Autodesk Inventor part; units mm, degrees
ref_plane "YZ Plane" through (0, 0, 0) normal (1, 0, 0) x (0, 1, 0)
ref_plane "XZ Plane" through (0, 0, 0) normal (0, 1, 0) x (-1, 0, 0)
ref_plane "XY Plane" through (0, 0, 0) normal (0, 0, 1) x (1, 0, 0)
sketch "Sketch1" plane through (0, 0, 0) normal (0, 0, 1) x (1, 0, 0)
  arc A0 (-18.1959, 74.3045) -> (-75.755, 10.6506) centre (0, 0) ccw
  line L0 (-78.9841, -12.3172) -> (-75.755, 10.6506)
  arc A1 (12.2439, 58.7374) -> (-59.4846, -7.8472) centre (0, 0) ccw
  line L1 (-18.1959, 74.3045) -> (9.302, 81.0383)
  line L2 (-59.4846, -7.8472) -> (-58.6652, -14.0586)
  line L3 (-78.9841, -12.3172) -> (-58.6652, -14.0586)
  line L4 (12.2439, 58.7374) -> (9.302, 81.0383)
  circle A2 centre (-67.5, 0) radius 3
  circle A3 centre (0, 67.5) radius 3
  circle A4 centre (52.0914, 68.8152) radius 17.05 construction
  line L5 (-32.9083, 50.1702) -> (-43.208, 63.1294) construction
  line L6 (-50.5977, 32.2471) -> (-61.3205, 45.7388) construction
  circle A5 centre (-61.4614, 29.8439) radius 2.5
  circle A6 centre (-29.2318, 61.6164) radius 2.5
  point P0 (0, 0)
  dimension "d2" = 25
  dimension "d3" = 5
  dimension "d4" = 5
  dimension "d6" = 10
extrude "Extrusion1" add sketch "Sketch1" along normal blind 4.4
properties part number "FrontMotorPlateBridge"
Geometry: final body of the model. Coordinates: model frame, mm. A direction names the side the tool comes from. Coordinates: 2 decimals unless noted, no trailing zeros. Order: outer loops, then holes, each group sorted by start corner. A loop starts at its lowest first (then second) coordinate and runs counter-clockwise, first axis right, second up. Notation, with made-up numbers: (-14.5, -7) -> (0.5, -7) arc R31 ccw to (0.5, 26) -> close; hole circle Ø10 at (77, -29). An arc over 180 degrees is marked (long way). Use CSV: the item, a comma, the result in double quotes.
1) Section B-B on x = 0. Output: boundary loops of the cut face in (y, z).
Findings:
outline,"(60, 0) -> (64.5, 0) -> (64.5, 4.4) -> (60, 4.4) -> close; (70.5, 0) -> (78.76, 0) -> (78.76, 4.4) -> (70.5, 4.4) -> close"
2) Section D-D on y = 49. Output: boundary loops of the cut face in (x, z).
Findings:
outline,"(-58.75, 0) -> (-34.63, 0) -> (-34.63, 4.4) -> (-58.75, 4.4) -> close"
3) Line query: line 1 (X direction, y = 1, z = 2.35); line 2 (Y direction, x = -68, z = 3.55); line 3 (Y direction, x = 2, z = 3.1). Output: solid intervals per line, ascending.
Findings:
line 1,"x = -77.11 to -70.33, -64.67 to -59.99"
line 2,"y = -13.26 to -2.96, 2.96 to 35.05"
line 3,"y = 59.97 to 65.26, 69.74 to 79.25"
4) Section A-A on y = 0. Output: boundary loops of the cut face in (x, z), then the cut area to 3 significant figures.
Findings:
outline,"(-77.25, 0) -> (-70.5, 0) -> (-70.5, 4.4) -> (-77.25, 4.4) -> close; (-64.5, 0) -> (-60, 0) -> (-60, 4.4) -> (-64.5, 4.4) -> close"
area,"49.5 mm^2"
5) Section C-C on z = 3.3. Output: boundary loops of the cut face in (x, y) (1 decimal).
Findings:
outline,"(-79, -12.3) -> (-58.7, -14.1) -> (-59.5, -7.8) arc R60 cw to (12.2, 58.7) -> (9.3, 81) -> (-18.2, 74.3) arc R76.5 ccw to (-75.8, 10.7) -> close; hole circle Ø6 at (-67.5, 0); hole circle Ø5 at (-61.5, 29.8); hole circle Ø5 at (-29.2, 61.6); hole circle Ø6 at (0, 67.5)"
6) Pin query (flat end, axial travel): pin 1 Ø5 at (x, y) = (-67.5, 0) entering from +Z; pin 2 Ø1.5 at (x, z) = (-10.5, 2.5) entering from +Y; pin 3 Ø2 at (y, z) = (60.5, 1) entering from +X. Return the tip coordinate at first contact, or that it passes through.
Findings:
pin 1,"passes through"
pin 2,"stops at y = 76.37"
pin 3,"stops at x = 12.14"
7) Mould query, pull axis Y, two halves, no side actions, for faces 1 (the flat face through (10.794, 69.732, 2.169)), 2 (the cylindrical face through (-0.65, 70.43, 2.17)), 3 (the flat face through (-68.967, -13.176, 2.169)), 4 (the flat face through (-44, 44, 4.4)). Classes: +Y half, -Y half, draft (parallel to the pull), parting line (faces both ways), or undercut.
Findings:
face 1,"+Y half"
face 2,"undercut"
face 3,"-Y half"
face 4,"draft"
8) Access query for faces 5 (the flat face through (-44, 44, 0)), 6 (the flat face through (-59.08, -10.91, 2.17)). Directions: +Z, -Z, +X, -X, +Y, -Y. A direction counts if a zero-diameter tool reaches every point of the face in a straight line with its end or side. Return the directions, or none.
Findings:
face 5,"-Z, +X, -X, +Y, -Y"
face 6,"+Z, -Z, +X"
